Geometry: final body of the model. Coordinates: model frame, mm. Face numbers are marked on the shaded views. Give positions to 0.01 mm unless a question says otherwise; leave off trailing zeros. Loops run counter-clockwise (first coordinate to the right, second up) from the corner with the lowest first, then second, coordinate; pieces in that order, holes last. Notation, with made-up numbers: (-37, -4) -> (-18, -4) arc R24 ccw to (-18, 10) -> close; hole circle Ø3 at (-21.75, -1). An arc over 180 degrees is marked (long way). Answer in a Markdown table with one row per item. Add a question column.
1) Section query A-A (z = 8.75). Return the cut outline in (x, y) (3 decimals).
2) Section query C-C (z = -7.75). Return the cut outline in (x, y) (3 decimals), plus the area to 3 significant figures.
3) Draft query along Z for the marked faces 1, 2 and 3. Return one class per face: +Z half, -Z half, draft (parallel to the pull), parting line (faces both ways), or undercut.
4) Line query: line 1 (Z direction, x = -7, y = -50); line 2 (Z direction, x = -51, y = -5); line 3 (Z direction, x = -54, y = -3.5). Output: solid intervals per line, ascending. Write a range as from..to.
5) First-contact query: P1, Ø10, axis at x = -18.5, z = 1.5, coming from the -Y side; P2, Ø5, axis at x = -8, z = -4, coming from the +Y side; P3, Ø4, axis at y = -27.5, z = -0.5, coming from the -X side. Flat tips, straight axial feed; report the tip coordinate or a pass-through.
```python
from build123d import *

# Parameters (mm, degrees)
SKETCH2_R           = 9.525
SKETCH3_R           = 11.1125
BOSS_EXTRUDE1_DEPTH = 3.175
SKETCH4_R           = 11.1125
BOSS_EXTRUDE2_DEPTH = 3.175
SKETCH5_R           = 6.35
CUT_EXTRUDE1_DEPTH  = 9.525
CUT_EXTRUDE1_DRAFT  = -5
SKETCH6_R           = 6.35
CUT_EXTRUDE2_DEPTH  = 9.525
CUT_EXTRUDE2_DRAFT  = -5


with BuildPart() as part:
    # Sweep2: sweep along a path in Sketch1
    with BuildLine(Plane.XY) as sweep2_path:
        ThreePointArc((-50.8, 0), (-35.921024484, -35.921024484), (0, -50.8))
    # Sketch2 → Sweep2 (sweep)
    with BuildSketch(Plane(origin=(0, 0, 0), x_dir=(1, 0, 0), z_dir=(0, 1, 0))):
        with Locations((-50.8, 0)):
            Circle(SKETCH2_R)
    sweep(path=sweep2_path.line)

    # Sketch3 → Boss-Extrude1 (add)
    with BuildSketch(Plane(origin=(0, 0, 0), x_dir=(1, 0, 0), z_dir=(0, 1, 0))):
        with Locations(Location((-50.8, 0, 0), (0, 0, 270))):
            Circle(SKETCH3_R)
    extrude(amount=BOSS_EXTRUDE1_DEPTH)

    # Sketch4 → Boss-Extrude2 (add)
    with BuildSketch(Plane(origin=(0, 0, 0), x_dir=(0, 0, -1), z_dir=(1, 0, 0))):
        with Locations(Location((0, -50.8, 0), (0, 0, 90))):
            Circle(SKETCH4_R)
    extrude(amount=BOSS_EXTRUDE2_DEPTH)


with BuildPart() as cut_extrude1_tool:
    # Sketch5 → Cut-Extrude1 (with draft: the straight prism first)
    with BuildSketch(Plane(origin=(0, 3.175, 0), x_dir=(1, 0, 0), z_dir=(0, 1, 0))):
        with Locations((-50.8, 0)):
            Circle(SKETCH5_R)
    extrude(amount=-CUT_EXTRUDE1_DEPTH)
    # Cut-Extrude1: the draft: its side faces are tilted about the plane it starts from
    cut_extrude1_sides = [cut_extrude1_tool.faces().sort_by_distance(p)[0] for p in [
        (-57.15, -1.5875, 0),
    ]]
    draft(cut_extrude1_sides, Plane(origin=(0, 3.175, 0), x_dir=(1, 0, 0), z_dir=(0, 1, 0)), CUT_EXTRUDE1_DRAFT)


with BuildPart() as part_1:
    add(part.part)

    # Cut-Extrude1: cut by cut_extrude1_tool
    add(cut_extrude1_tool.part, mode=Mode.SUBTRACT)


with BuildPart() as cut_extrude2_tool:
    # Sketch6 → Cut-Extrude2 (with draft: the straight prism first)
    with BuildSketch(Plane(origin=(3.175, 0, 0), x_dir=(0, 0, -1), z_dir=(1, 0, 0))):
        with Locations((0, -50.8)):
            Circle(SKETCH6_R)
    extrude(amount=-CUT_EXTRUDE2_DEPTH)
    # Cut-Extrude2: the draft: its side faces are tilted about the plane it starts from
    cut_extrude2_sides = [cut_extrude2_tool.faces().sort_by_distance(p)[0] for p in [
        (-1.5875, -50.8, 6.35),
    ]]
    draft(cut_extrude2_sides, Plane(origin=(3.175, 0, 0), x_dir=(0, 0, -1), z_dir=(1, 0, 0)), CUT_EXTRUDE2_DRAFT)


with BuildPart() as part_2:
    add(part_1.part)

    # Cut-Extrude2: cut by cut_extrude2_tool
    add(cut_extrude2_tool.part, mode=Mode.SUBTRACT)


solid = part_2.part
```
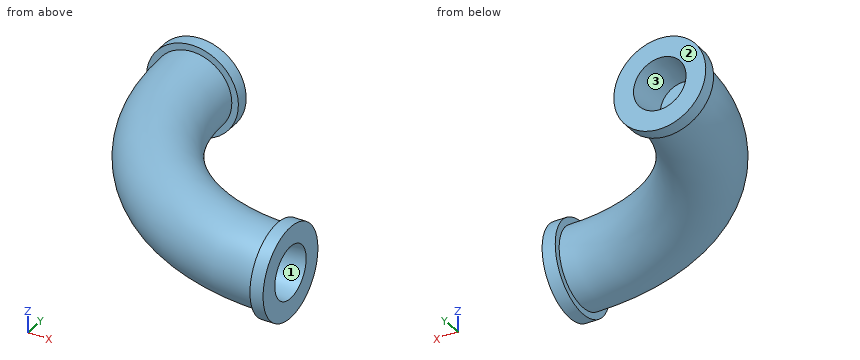
Evaluation:
| question | item | result |
|---|---|---|
| 1 | outline | (-57.65, 0) -> (-54.563, 0) arc R54.563 ccw to (0, -54.563) -> (0, -57.65) -> (3.175, -57.65) -> (3.175, -43.95) -> (0, -43.95) -> (0, -47.037) arc R47.037 cw to (-47.037, 0) -> (-43.95, 0) -> (-43.95, 3.175) -> (-57.65, 3.175) -> close |
| 2 | outline | (-58.764, 0) -> (-56.337, 0) arc R56.337 ccw to (0, -56.337) -> (0, -58.764) -> (3.175, -58.764) -> (3.175, -42.836) -> (0, -42.836) -> (0, -45.263) arc R45.263 cw to (-45.263, 0) -> (-42.836, 0) -> (-42.836, 3.175) -> (-58.764, 3.175) -> close |
| 2 | area | 985 mm² |
| 3 | face 1 | undercut |
| 3 | face 2 | draft |
| 3 | face 3 | undercut |
| 4 | line 1 | -9.52..9.52 |
| 4 | line 2 | -9.51..-5.63, 5.63..9.51 |
| 4 | line 3 | -8.93..-4.8, 4.8..8.93 |
| 5 | P1 | y = -58.76 |
| 5 | P2 | y = -40.38 |
| 5 | P3 | x = -54.66 |
